from build123d import *

# Parameters (mm, degrees)
F0_R      = 3.175
F1_DEPTH  = 152.4
F2_R      = 6.35
F3_DEPTH  = 2.54
F4_R      = 3.175
F5_DEPTH  = 25.4
F6_R      = 9.525
F7_DEPTH  = 19.05
F8_SIZE   = 5.08
F10_D     = 1.27
F10_DEPTH = 25.4
F10_TIP   = 0.3815464931


with BuildPart() as f1:
    # F0 (on Top) → F1 (new body)
    with BuildSketch(Plane.XY):
        Circle(F0_R)
    extrude(amount=F1_DEPTH)

    # F2 (on face) → F3 (join)
    with BuildSketch(Plane(origin=(0, 0, 0), x_dir=(1, 0, 0), z_dir=(0, 0, -1))):
        Circle(F2_R)
    extrude(amount=F3_DEPTH)

    # F4 (on face) → F5 (join)
    with BuildSketch(Plane(origin=(0, 0, -2.54), x_dir=(1, 0, 0), z_dir=(0, 0, -1))):
        Circle(F4_R)
    extrude(amount=F5_DEPTH)

    # F6 (on face) → F7 (join)
    with BuildSketch(Plane(origin=(0, 0, -27.94), x_dir=(1, 0, 0), z_dir=(0, 0, -1))):
        Circle(F6_R)
    extrude(amount=F7_DEPTH)

    # F8
    f8_edges = [f1.edges().sort_by_distance(p)[0] for p in [
        (-9.525, 0, -46.99),
    ]]
    chamfer(f8_edges, length=F8_SIZE)

    # F10
    with Locations(Plane.XY.offset(152.4)):
        with Locations((0, 0)):
            Hole(F10_D / 2, depth=F10_DEPTH)
            with Locations((0, 0, -(F10_DEPTH + F10_TIP / 2))):  # 118° drill point
                Cone(0, F10_D / 2, F10_TIP, mode=Mode.SUBTRACT)


solid = f1.part
The model under review builds one solid part; all positions refer to its coordinate system, in mm. A direction names the side the tool comes from. Round coordinates to 2 decimals unless told otherwise and drop trailing zeros. Order: outer loops, then holes, each group sorted by start corner. A loop starts at its lowest first (then second) coordinate and runs counter-clockwise, first axis right, second up. Notation, with made-up numbers: (60, 77) -> (103, 77) arc R20 ccw to (103, 86) -> close; hole circle Ø4 at (9.25, -24.5). An arc over 180 degrees is marked (long way). Write item = value, one per line. Start each with the question number.
Item 1: Consider section A-A on z = 104. Write out the cut boundary in (x, y) (3 decimals).
Item 2: Clearance check with flat-ended pins moving along their axes: pin 1 Ø1 at (x, z) = (0.5, 118.5) entering from -Y (3 decimals); pin 2 Ø0.8 at (x, y) = (0, 0) entering from +Z; pin 3 Ø4 at (x, z) = (-4, 88) entering from +Y. State where each tip first meets the part, or that it passes through.
Item 3: For faces 5 (the face through (-0.69, -3.1, 75.13)), 6 (the face through (-7.559, 5.796, -34.827)), 7 (the face through (-2, -3, -2.54)), list the 3-axis set-ups (+Z, -Z, +X, -X, +Y, -Y) from which the entire face can be reached by the end or side of a thin tool; tool diameter is ignored.
Item 4: For line 1 along Y through (x, z) = (0, 139) (3 decimals); line 2 along Z through (x, y) = (1.25, -4); line 3 along Y through (x, z) = (-0.5, 74.5), list the stretches that pass through material, from the lowest coordinate up.
Item 5: Mouldability with a two-part tool opening along Z and no side actions: class faces 1 (the face through (4, 0, -27.94)), 2 (the face through (1, 0, 152.4)), 3 (the face through (-1.02, 4.58, -46.74)), 4 (the face through (-0.69, 3.1, -15.06)) as released by +Z, released by -Z, zero draft, split by the parting line, or undercut.
Item 6: Consider section B-B on z = -32.5. Write out the cut boundary in (x, y) (3 decimals), plus the area to 3 significant figures.
Conclusion:
q1.outline = circle Ø6.35 at (0, 0)
q2.pin_1 = -3.175
q2.pin_2 = 126.86
q2.pin_3 = 2.47
q3.face_5 = +Z
q3.face_6 = +Z, -Z
q3.face_7 = none
q4.line_1 = -3.175 to -0.635, 0.635 to 3.175
q4.line_2 = -46.99 to -27.94, -2.54 to 0
q4.line_3 = -3.14 to 3.14
q5.face_1 = undercut
q5.face_2 = released by +Z
q5.face_3 = released by -Z
q5.face_4 = undercut
q6.outline = circle Ø19.05 at (0, 0)
q6.area = 285 mm2
